```python
from build123d import *

# Parameters (mm, degrees)
SKETCH5_W            = 110
SKETCH5_H            = 80
BOSS_EXTRUDE8_DEPTH  = 2
SKETCH9_R            = 3.5
BOSS_EXTRUDE11_DEPTH = 7
SKETCH11_R           = 1.5
CUT_EXTRUDE1_DEPTH   = 7
SKETCH12_W           = 110
SKETCH12_H           = 80
SKETCH12_W_2         = 106
SKETCH12_H_2         = 76
BOSS_EXTRUDE12_DEPTH = 29
BOSS_EXTRUDE14_DEPTH = 7
BOSS_EXTRUDE15_DEPTH = 7
CUT_EXTRUDE2_REACH   = 112
SKETCH16_W           = 40
SKETCH16_H           = 21
BOSS_EXTRUDE16_DEPTH = 7
BOSS_EXTRUDE17_DEPTH = 7
BOSS_EXTRUDE18_DEPTH = 40
CUT_EXTRUDE4_REACH   = 112
SKETCH23_R           = 1.25
CUT_EXTRUDE5_REACH   = 112
SKETCH24_R           = 1.25


with BuildPart() as part:
    # Sketch5 → Boss-Extrude8 (new body)
    with BuildSketch(Plane(origin=(0, 0, 0), x_dir=(1, 0, 0), z_dir=(0, 1, 0))):
        with Locations((-25, 43.57615894)):
            Rectangle(SKETCH5_W, SKETCH5_H)
    extrude(amount=BOSS_EXTRUDE8_DEPTH)

    # Sketch9 → Boss-Extrude11 (add)
    with BuildSketch(Plane(origin=(0, 2, 0), x_dir=(1, 0, 0), z_dir=(0, 1, 0))):
        with Locations((-74, 15.57615894)):
            Circle(SKETCH9_R)
        with Locations((-74, 71.57615894)):
            Circle(SKETCH9_R)
        with Locations((15, 15.57615894)):
            Circle(SKETCH9_R)
        with Locations((15, 71.57615894)):
            Circle(SKETCH9_R)
    extrude(amount=BOSS_EXTRUDE11_DEPTH)

    # Sketch11 → Cut-Extrude1 (cut)
    with BuildSketch(Plane(origin=(0, 9, 0), x_dir=(1, 0, 0), z_dir=(0, 1, 0))):
        with Locations((-74, 15.57615894)):
            Circle(SKETCH11_R)
        with Locations((-74, 71.405276361)):
            Circle(SKETCH11_R)
        with Locations((15, 71.57615894)):
            Circle(SKETCH11_R)
        with Locations((15, 15.57615894)):
            Circle(SKETCH11_R)
    extrude(amount=-CUT_EXTRUDE1_DEPTH, mode=Mode.SUBTRACT)

    # Sketch12 → Boss-Extrude12 (add)
    with BuildSketch(Plane(origin=(0, 2, 0), x_dir=(1, 0, 0), z_dir=(0, 1, 0))):
        with Locations((-25, 43.57615894)):
            Rectangle(SKETCH12_W, SKETCH12_H)
        with Locations((-25, 43.57615894)):
            Rectangle(SKETCH12_W_2, SKETCH12_H_2, mode=Mode.SUBTRACT)
    extrude(amount=BOSS_EXTRUDE12_DEPTH)

    # Sketch14 → Boss-Extrude14 (add)
    with BuildSketch(Plane(origin=(0, 2, 0), x_dir=(1, 0, 0), z_dir=(0, 1, 0))):
        Polygon((-74, 12.07615894), (-78, 12.07615894), (-78, 19.07615894), (-74, 19.07615894), (-77.5, 15.57615894), align=None)
    extrude(amount=BOSS_EXTRUDE14_DEPTH)

    # Sketch15 → Boss-Extrude15 (add)
    with BuildSketch(Plane(origin=(0, 2, 0), x_dir=(1, 0, 0), z_dir=(0, 1, 0))):
        Polygon((-74, 75.07615894), (-78, 75.07615894), (-78, 68.07615894), (-74, 68.07615894), (-77.5, 71.57615894), align=None)
    extrude(amount=BOSS_EXTRUDE15_DEPTH)

    # Sketch16 → Cut-Extrude2 (cut, up to next)
    with BuildSketch(Plane(origin=(30, 0, 0), x_dir=(0, 0, -1), z_dir=(1, 0, 0)), mode=Mode.PRIVATE) as cut_extrude2_sk1:
        with Locations((43.57615894, 20.5)):
            Rectangle(SKETCH16_W, SKETCH16_H)
    cut_extrude2_tool1 = extrude(cut_extrude2_sk1.sketch, amount=-CUT_EXTRUDE2_REACH, mode=Mode.PRIVATE) & part.part
    add(cut_extrude2_tool1.solids().sort_by_distance((30, 20.5, -43.576159))[0], mode=Mode.SUBTRACT)

    # Sketch17 → Boss-Extrude16 (add)
    with BuildSketch(Plane(origin=(0, 2, 0), x_dir=(1, 0, 0), z_dir=(0, 1, 0))):
        Polygon((15, 75.07615894), (28, 75.07615894), (28, 68.07615894), (15, 68.07615894), (18.5, 71.57615894), align=None)
    extrude(amount=BOSS_EXTRUDE16_DEPTH)

    # Sketch18 → Boss-Extrude17 (add)
    with BuildSketch(Plane(origin=(0, 2, 0), x_dir=(1, 0, 0), z_dir=(0, 1, 0))):
        Polygon((15, 19.07615894), (28, 19.07615894), (28, 12.07615894), (15, 12.07615894), (18.5, 15.57615894), align=None)
    extrude(amount=BOSS_EXTRUDE17_DEPTH)

    # Sketch22 → Boss-Extrude18 (add)
    with BuildSketch(Plane.XY.offset(-63.57615894)):
        Polygon((30, 10), (35, 10), (30, 0), align=None)
    extrude(amount=BOSS_EXTRUDE18_DEPTH)

    # Sketch23 → Cut-Extrude4 (cut, up to next)
    with BuildSketch(Plane(origin=(30, 0, 0), x_dir=(0, 0, -1), z_dir=(1, 0, 0)), mode=Mode.PRIVATE) as cut_extrude4_sk1:
        with Locations((10.57615894, 7)):
            Circle(SKETCH23_R)
    cut_extrude4_tool1 = extrude(cut_extrude4_sk1.sketch, amount=-CUT_EXTRUDE4_REACH, mode=Mode.PRIVATE) & part.part
    add(cut_extrude4_tool1.solids().sort_by_distance((30, 7, -10.576159))[0], mode=Mode.SUBTRACT)

    # Sketch24 → Cut-Extrude5 (cut, up to next)
    with BuildSketch(Plane(origin=(30, 0, 0), x_dir=(0, 0, -1), z_dir=(1, 0, 0)), mode=Mode.PRIVATE) as cut_extrude5_sk1:
        with Locations((76.57615894, 7)):
            Circle(SKETCH24_R)
    cut_extrude5_tool1 = extrude(cut_extrude5_sk1.sketch, amount=-CUT_EXTRUDE5_REACH, mode=Mode.PRIVATE) & part.part
    add(cut_extrude5_tool1.solids().sort_by_distance((30, 7, -76.576159))[0], mode=Mode.SUBTRACT)


solid = part.part
```
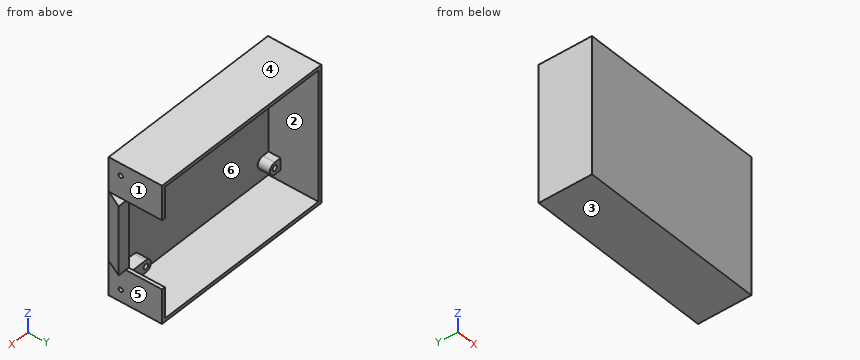
Can you work these out from the model? Positions are in its coordinate system, mm. Face numbers are marked on the shaded views. A direction names the side the tool comes from. Give positions to 0.01 mm unless a question says otherwise; leave off trailing zeros. Order: outer loops, then holes, each group sorted by start corner. A loop starts at its lowest first (then second) coordinate and runs counter-clockwise, first axis right, second up. Notation, with made-up numbers: M 60.5,-39.5 L 88.5,-39.5 A33 cw 88.5,-6.5 Z; hole C 14.25,55 d10. An arc over 180 degrees is marked long. Write item = value, one per line. Start each with the question number.
Q1. Will these pins go through, and if not, where does the flat tip stop? pin 1 Ø23 at (x, z) = (-49.5, -27) entering from +Y; pin 2 Ø2 at (x, z) = (32.5, -46) entering from +Y; pin 3 Ø10 at (y, z) = (21.5, -9.5) entering from +X.
Q2. We'd pull the mould along Z, two halves only. Please class the marked faces 4, 5 and 6: pulls with the +Z half, pulls with the -Z half, needs draft (parallel to the pull), parting line crosses it, or undercut.
Q3. For the marked faces 1, 2 and 3, which set-ups out of +Z, -Z, +X, -X, +Y, -Y let a thin tool reach every point of the face, with its end or its side?
Q4. Suppose I cut it at D-D (y = 7). Count the separate pieces of the cut face and the enclosed holes in it, plus the area to 3 significant figures.
Q5. Suppose I cut it at C-C (z = -55). Write out the boundary of the cut face in (x, y), plus the area to 3 significant figures.
Q6. I need wall thicknesses on probe 1 along Z at (x, y) = (15, 6.25); probe 2 along Z at (x, y) = (-74, 4); probe 3 along Z at (x, y) = (5.5, 7). Which ranges of each line are inside material? Lowest first, please. Write a range as [from, to].
Q7. Suppose I cut it at B-B (x = -3). Write out the boundary of the cut face in (y, z).
Q8. Suppose I cut it at A-A (y = 14.5). Write out the boundary of the cut face in (x, z).
Check result:
q1.pin_1 = 2
q1.pin_2 = 10
q1.pin_3 = 30
q2.face_4 = pulls with the +Z half
q2.face_5 = needs draft
q2.face_6 = undercut
q3.face_1 = +Z, +X, +Y, -Y
q3.face_2 = +Y
q3.face_3 = -Z, +X, -X, +Y, -Y
q4.separate_pieces = 2
q4.enclosed_holes = 4
q4.area = 1,160 mm2
q5.outline = M -80,0 L 30,0 L 35,10 L 28,10 L 28,2 L -78,2 L -78,31 L -80,31 Z
q5.area = 319 mm2
q6.probe_1 = [-83.58, -81.58], [-75.08, -73.08], [-70.08, -68.08], [-19.08, -17.08], [-14.08, -12.08], [-5.58, -3.58]
q6.probe_2 = [-83.58, -81.58], [-75.08, -72.91], [-69.91, -68.08], [-19.08, -17.08], [-14.08, -12.08], [-5.58, -3.58]
q6.probe_3 = [-83.58, -81.58], [-5.58, -3.58]
q7.outline = M 0,-83.58 L 31,-83.58 L 31,-81.58 L 2,-81.58 L 2,-5.58 L 31,-5.58 L 31,-3.58 L 0,-3.58 Z
q8.outline = M -80,-83.58 L 30,-83.58 L 30,-63.58 L 28,-63.58 L 28,-81.58 L -78,-81.58 L -78,-5.58 L 28,-5.58 L 28,-23.58 L 30,-23.58 L 30,-3.58 L -80,-3.58 Z
